Autodesk Inventor part; units mm, degrees
ref_plane "YZ Plane" through (0, 0, 0) normal (1, 0, 0) x (0, 1, 0)
ref_plane "XZ Plane" through (0, 0, 0) normal (0, 1, 0) x (-1, 0, 0)
ref_plane "XY Plane" through (0, 0, 0) normal (0, 0, 1) x (1, 0, 0)
sketch "Sketch1" plane through (0, 0, 0) normal (0, 1, 0) x (-1, 0, 0)
  line L0 (24, 138) -> (-24, 138)
  line L1 (-24, 138) -> (-24, -138)
  line L2 (-24, -138) -> (24, -138)
  line L3 (24, -138) -> (24, 138)
  point P0 (0, 0)
  dimension "d0" = 48
  dimension "d1" = 276
extrude "Extrusion1" add sketch "Sketch1" along normal blind 3
sketch "Sketch2" plane through (0, 3, 0) normal (0, 1, 0) x (1, 0, 0)
  line L0 (-24, 138) -> (-24, -138)
  line L1 (-24, -138) -> (-21, -138)
  line L2 (-21, -138) -> (-21, -90)
  line L3 (-21, -90) -> (-24, -90)
  line L4 (-24, -90) -> (-24, -138)
  line L5 (24, -138) -> (24, 138)
  line L6 (-21, -90) -> (24, -90)
  line L7 (24, -90) -> (24, -93)
  line L8 (24, -93) -> (-21, -93)
  line L9 (-21, -93) -> (-21, -90)
  line L10 (-24, -138) -> (24, -138)
  line L11 (24, -93) -> (21, -93)
  line L12 (21, -93) -> (21, -138)
  line L13 (21, -138) -> (24, -138)
  line L14 (24, -138) -> (24, -93)
  line L15 (21, -138) -> (-21, -138)
  line L16 (-21, -138) -> (-21, -135)
  line L17 (-21, -135) -> (21, -135)
  line L18 (21, -135) -> (21, -138)
  point P0 (0, 0)
  dimension "d4" = 3
  dimension "d5" = 48
  dimension "d6" = 3
  dimension "d7" = 3
  dimension "d8" = 3
extrude "Extrusion2" add sketch "Sketch2" along normal blind 3 contours L3 L2 L1 L0 | L6 L5 L8 L2 | L2 L17 L12 L10 | L12 L8 L5 L10
mirror "Mirror1" about plane through (0, 0, 0) normal (0, 0, 1) of "Extrusion2"
sketch "Sketch3" plane through (0, 0, 0) normal (0, -1, 0) x (1, 0, 0)
  line L0 (24, -90) -> (-24, -90)
  line L1 (24, 138) -> (24, -138)
  line L2 (-24, -90) -> (24, -90)
  line L3 (24, -90) -> (24, -93)
  line L4 (24, -93) -> (-24, -93)
  line L5 (-24, -93) -> (-24, -90)
  line L6 (-24, 90) -> (24, 90)
  line L7 (24, 90) -> (21, 90)
  line L8 (21, 90) -> (21, -90)
  line L9 (21, -90) -> (24, -90)
  line L10 (24, -90) -> (24, 90)
  line L11 (-24, 90) -> (24, 90)
  line L12 (24, 90) -> (24, 93)
  line L13 (24, 93) -> (-24, 93)
  line L14 (-24, 93) -> (-24, 90)
  point P0 (0, 0)
  dimension "d11" = 3
  dimension "d12" = 3
  dimension "d13" = 3
extrude "Extrusion3" add sketch "Sketch3" along normal blind 35
sketch "Sketch4" plane through (-24, 0, -90) normal (0, 0, 1) x (1, 0, 0)
  line L0 (0, -35) -> (45, -35)
  line L1 (45, 0) -> (45, -35)
  line L2 (0, -35) -> (45, -35)
  line L3 (45, -35) -> (45, -31)
  line L4 (45, -31) -> (0, -31)
  line L5 (0, -31) -> (0, -35)
  point P0 (24, 0)
  dimension "d16" = 4
extrude "Extrusion4" add sketch "Sketch4" along normal blind 8
sketch "Sketch5" plane through (-24, -31, -90) normal (0, 1, 0) x (1, 0, 0)
  line L0 (0, -8) -> (45, -8)
  line L1 (45, 0) -> (45, -8)
  line L2 (0, -8) -> (45, -8)
  line L3 (45, -8) -> (45, -4)
  line L4 (45, -4) -> (0, -4)
  line L5 (0, -4) -> (0, -8)
  point P0 (24, -90)
  dimension "d19" = 4
extrude "Extrusion5" add sketch "Sketch5" along normal blind 4
sketch "Sketch6" plane through (0, 0, 0) normal (0, -1, 0) x (1, 0, 0)
  line L0 (21, -86) -> (-24, -86)
  line L1 (-24, -82) -> (21, -82)
  line L2 (21, -82) -> (21, -86)
  line L3 (21, -86) -> (-24, -86)
  line L4 (-24, -86) -> (-24, -82)
  point P0 (0, 0)
  dimension "d22" = 4
extrude "Extrusion6" add sketch "Sketch6" along normal blind 4
mirror "Mirror2" about plane through (0, 0, 0) normal (0, 0, 1) of "Extrusion6", "Extrusion5", "Extrusion4"
sketch "Sketch7" plane through (0, 0, 0) normal (0, -1, 0) x (1, 0, 0)
  circle A0 centre (-15, -129) radius 3
  circle A1 centre (15, -129) radius 3
  circle A2 centre (15, -99) radius 3
  circle A3 centre (-15, -99) radius 3
  point P0 (0, 0)
  dimension "d25" = 6
  dimension "d26" = 6
  dimension "d27" = 6
  dimension "d28" = 6
extrude "Extrusion7" cut sketch "Sketch7" against normal blind 4
mirror "Mirror3" about plane through (0, 0, 0) normal (0, 0, 1) of "Extrusion7"
sketch "Sketch8" plane through (0, 0, 0) normal (0, -1, 0) x (1, 0, 0)
  line L0 (21, 82) -> (21, -82)
  line L1 (-24, -82) -> (-24, 82)
  line L2 (21, -20) -> (-24, -20)
  line L3 (-24, -20) -> (-24, -17)
  line L4 (-24, -17) -> (21, -17)
  line L5 (21, -17) -> (21, -20)
  point P0 (0, 0)
  dimension "d31" = 3
extrude "Extrusion8" add sketch "Sketch8" along normal blind 42.3
sketch "Sketch9" plane through (21, 0, -20) normal (0, 0, -1) x (-1, 0, 0)
  circle A0 centre (39.35, -5.65) radius 4
  circle A1 centre (39.35, -36.65) radius 4
  circle A2 centre (8.35, -5.65) radius 4
  circle A3 centre (8.35, -36.65) radius 4
  point P0 (21, 0)
  dimension "d34" = 8
  dimension "d35" = 8
  dimension "d36" = 8
  dimension "d37" = 8
extrude "Extrusion9" add sketch "Sketch9" along normal blind 3
sketch "Sketch10" plane through (-18.35, -36.65, -23) normal (0, 0, -1) x (-1, 0, 0)
  circle A0 centre (0, 0) radius 3
  circle A1 centre (0, 31) radius 4
  circle A2 centre (0, 31) radius 3
  circle A3 centre (-31, 0) radius 4
  circle A4 centre (-31, 0) radius 3
  circle A5 centre (-31, 31) radius 4
  circle A6 centre (-31, 31) radius 3
  point P0 (-18.35, 36.65)
  dimension "d40" = 6
  dimension "d41" = 6
  dimension "d42" = 6
  dimension "d43" = 6
extrude "Extrusion10" cut sketch "Sketch10" against normal blind 2 contours A0 | A2 | A4 | A6
sketch "Sketch11" plane through (21, 0, -20) normal (0, 0, -1) x (-1, 0, 0)
  circle A0 centre (23.85, -21.15) radius 12.5
  circle A1 centre (39.35, -36.65) radius 3
  circle A2 centre (39.35, -36.65) radius 2
  circle A3 centre (8.35, -36.65) radius 3
  circle A4 centre (8.35, -36.65) radius 2
  circle A5 centre (8.35, -5.65) radius 4
  circle A6 centre (8.35, -5.65) radius 2
  circle A7 centre (39.35, -5.65) radius 4
  circle A8 centre (39.35, -5.65) radius 2
  point P0 (21, 0)
  dimension "d46" = 25
  dimension "d47" = 4
  dimension "d48" = 4
  dimension "d49" = 4
  dimension "d50" = 4
extrude "Extrusion11" cut sketch "Sketch11" along normal mid plane 10 contours A0 | A2 | A4 | A6 | A8
properties part number "carriageEnd"
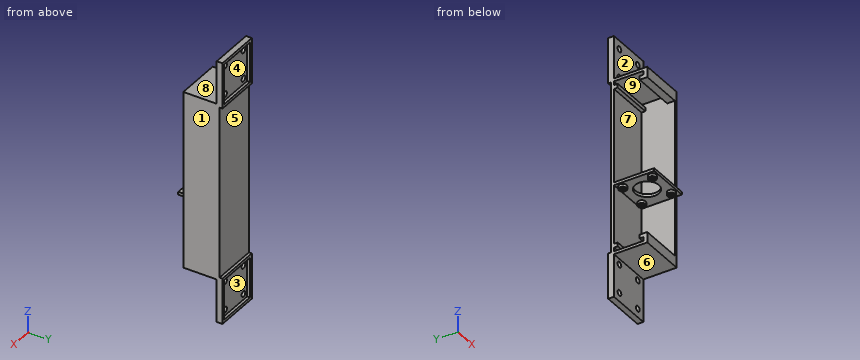
The listing builds one solid part. Answer for the finished solid, in the listing's coordinates (mm). Face numbers are marked on the shaded views. A direction names the side the tool comes from. Round coordinates to 2 decimals unless told otherwise and drop trailing zeros. Loops run counter-clockwise (first coordinate to the right, second up) from the corner with the lowest first, then second, coordinate; pieces in that order, holes last.
1) Given P1, Ø8, axis at x = -14.5, z = 26, coming from the -Y side; P2, Ø12, axis at x = 10.5, y = -32, coming from the -Z side; P3, Ø6, axis at x = -15.5, y = -14, coming from the +Z side; P4, Ø4, axis at x = 18.5, z = -16, coming from the -Y side, each flat-ended and moving along its own axis, determine where each tip first touches the part or whether it passes through.
Outcome:
P1: stops at y = 0
P2: stops at z = -93
P3: stops at z = 93
P4: stops at y = -42.3
2) Consider line 1 (Z direction, x = -22, y = -1); line 2 (Z direction, x = 15, y = 1.2); line 3 (Y direction, x = -18.35, z = -19.45). Determine where each line is inside the solid, lowest interval first.
Outcome:
line 1: z = -93 to -90, -86 to -82, -20 to -17, 82 to 86, 90 to 93
line 2: z = -138 to -132, -126 to -102, -96 to 96, 102 to 126, 132 to 138
line 3: y = -42.3 to -38.65, -34.65 to -7.65, -3.65 to 3
3) For a pull along X with two mould halves and no side action, classify the marked faces 1, 2, 3 and 4 as released by +X, released by -X, zero draft, split by the parting line, or undercut.
Outcome:
face 1: released by +X
face 2: zero draft
face 3: undercut
face 4: undercut
4) A cutting plane is placed at A-A on z = 99. Determine the outline of the cut face in (x, y), plus the area to 3 significant figures.
Outcome:
outline: (-24, 0) - (-18, 0) - (-18, 3) - (-21, 3) - (-21, 6) - (-24, 6) - close; (-12, 0) - (12, 0) - (12, 3) - (-12, 3) - close; (18, 0) - (24, 0) - (24, 6) - (21, 6) - (21, 3) - (18, 3) - close
area: 126 mm2
5) For the marked faces 5, 6, 7, 8 and 9, determine the directions among +Z, -Z, +X, -X, +Y, -Y from which every point of the face is accessible in a straight line to the end or side of a thin tool.
Outcome:
face 5: +X, -X, +Y
face 6: -Z, +X, -X, -Y
face 7: -X, -Y
face 8: +Z, +X, -X, -Y
face 9: -X
6) A cutting plane is placed at B-B on z = 69.5. Determine the outline of the cut face in (x, y).
Outcome:
outline: (-24, 0) - (21, 0) - (21, -35) - (24, -35) - (24, 3) - (-24, 3) - close
